Input: part model. Units: mm. Frame: model coordinates. Round coordinates to 2 decimals unless told otherwise and drop trailing zeros. Loops run counter-clockwise (first coordinate to the right, second up) from the corner with the lowest first, then second, coordinate; pieces in that order, holes last. Notation, with made-up numbers: M 18.25,7.25 L 53.25,7.25 A5 cw 53.25,11.25 Z; hole C 34.5,85.5 d4. An arc over 180 degrees is marked long. Put each result on its own line as item: value. Start each with the question number.
1) Section D-D on z = 23.5. Output: boundary loops of the cut face in (x, y), plus the area to 3 significant figures.
2) Draft query along X for faces 1 (the face through (25.007, -12.522, 13.449)), 2 (the face through (12, -25.4, 14)), 3 (the face through (19.484, -13, 2)). Return one class per face: +X half, -X half, draft (parallel to the pull), parting line (faces both ways), or undercut.
3) Line query: probe 1 along Z at (x, y) = (6.5, -17.5); probe 2 along X at (y, z) = (-5.5, 19.25); probe 3 along X at (y, z) = (-6, 22.5). Output: solid intervals per line, ascending.
4) Section A-A on y = -20. Output: boundary loops of the cut face in (x, z).
5) Section C-C on x = 10.5. Output: boundary loops of the cut face in (y, z).
6) Section B-B on z = 1.5. Output: boundary loops of the cut face in (x, y), plus the area to 3 significant figures.
7) Pin query (flat end, axial travel): pin 1 (3 mm diameter, centred on y = -16, z = 3, fed in from -X); pin 2 (8 mm diameter, centred on y = -5.5, z = 3.5, fed in from +X); pin 3 (7 mm diameter, centred on y = -14.5, z = 1, fed in from -X). Return the tip coordinate at first contact, or that it passes through.
from build123d import *

# Parameters (mm, degrees)
F1_DEPTH = 25.4
F3_DEPTH = 25.4
F4_DEPTH = 50.8


with BuildPart() as f1:
    # F0 (on Front) → F1 (new body)
    with BuildSketch(Plane.XZ):
        Polygon((6.2624249645, 28.3681909489), (-7.2102827521, -0.3815681245), (30.8836984568, -1.0587650323), (18.9624249645, 28.3681909489), align=None)
    extrude(amount=F1_DEPTH)

    # F2 (on face) → F3 (join)
    with BuildSketch(Plane.XZ.offset(25.4)):
        Polygon((6.7862393458, 5.7196156272), (6.6733910244, -0.6283782675), (19.4842330822, -0.8561166753), (19.4842330822, 5.4938833247), align=None)
    extrude(amount=F3_DEPTH)

    # F4 (cut): a face of the model
    f4_faces = [f1.faces().sort_by_distance(p)[0] for p in [
        (13.1069825312, -50.8, 2.42756979),
    ]]
    extrude(f4_faces, amount=-F4_DEPTH, mode=Mode.SUBTRACT)


solid = f1.part
Geometry results:
1. outline: M 3.98,-25.4 L 20.93,-25.4 L 20.93,0 L 3.98,0 Z
1. area: 431 mm²
2. face 1: +X half
2. face 2: draft
2. face 3: undercut
3. probe 1: z = -0.63 to 28.37
3. probe 2: x = 1.99 to 22.66
3. probe 3: x = 3.51 to 21.34
4. outline: M -7.21,-0.38 L 6.67,-0.63 L 6.79,5.72 L 19.48,5.49 L 19.48,-0.86 L 30.88,-1.06 L 18.96,28.37 L 6.26,28.37 Z
5. outline: M -25.4,5.65 L 0,5.65 L 0,28.37 L -25.4,28.37 Z
6. outline: M -6.33,-25.4 L 6.71,-25.4 L 6.71,0 L -6.33,0 Z; M 19.48,-25.4 L 29.85,-25.4 L 29.85,0 L 19.48,0 Z
6. area: 594 mm²
7. pin 1: stops at x = -6.33
7. pin 2: stops at x = 30.66
7. pin 3: stops at x = -7.21
